from build123d import *

# Parameters (mm, degrees)
SKETCH_1_W          = 16
SKETCH_1_H          = 26
EXTRUDE_1_DEPTH     = 5
CUT_EXTRUDE_START   = 1
SKETCH_2_W          = 14
SKETCH_2_H          = 25
CUT_EXTRUDE_1_DEPTH = 10
EXTRUDE_START       = 5
SKETCH_3_W          = 16
SKETCH_3_H          = 26
EXTRUDE_3_DEPTH     = 1
CUT_EXTRUDE_START_2 = 6
SKETCH_4_W          = 14
SKETCH_4_H          = 17
CUT_EXTRUDE_2_DEPTH = 1
SKETCH_6_W          = 16
SKETCH_6_H          = 26
CUT_EXTRUDE_4_DEPTH = 5


with BuildPart() as part:
    # 스케치1 → 보스-돌출1 (new body)
    with BuildSketch(Plane(origin=(0, 0, 0), x_dir=(1, 0, 0), z_dir=(0, 1, 0))):
        Rectangle(SKETCH_1_W, SKETCH_1_H)
    extrude(amount=EXTRUDE_1_DEPTH)

    # 스케치2 → 컷-돌출1 (cut)
    with BuildSketch(Plane(origin=(0, 0, 0), x_dir=(1, 0, 0), z_dir=(0, 1, 0)).offset(CUT_EXTRUDE_START)):
        with Locations((0, 0.5)):
            Rectangle(SKETCH_2_W, SKETCH_2_H)
    extrude(amount=CUT_EXTRUDE_1_DEPTH, mode=Mode.SUBTRACT)

    # 스케치6 → 컷-돌출4 (cut)
    with BuildSketch(Plane.XZ):
        Rectangle(SKETCH_6_W, SKETCH_6_H)
    extrude(amount=-CUT_EXTRUDE_4_DEPTH, mode=Mode.SUBTRACT)


with BuildPart() as body_2:
    # 스케치3 → 보스-돌출3 (new body)
    with BuildSketch(Plane(origin=(0, 0, 0), x_dir=(1, 0, 0), z_dir=(0, 1, 0)).offset(EXTRUDE_START)):
        Rectangle(SKETCH_3_W, SKETCH_3_H)
    extrude(amount=EXTRUDE_3_DEPTH)

    # 스케치4 → 컷-돌출2 (cut)
    with BuildSketch(Plane(origin=(0, 0, 0), x_dir=(1, 0, 0), z_dir=(0, 1, 0)).offset(CUT_EXTRUDE_START_2)):
        with Locations((0, -1.5)):
            Rectangle(SKETCH_4_W, SKETCH_4_H)
    extrude(amount=-CUT_EXTRUDE_2_DEPTH, mode=Mode.SUBTRACT)


solid = body_2.part
For this review, take the finished solid that the model builds, in its own axes (mm). A direction names the side the tool comes from. Round coordinates to 2 decimals unless told otherwise and drop trailing zeros. Order: outer loops, then holes, each group sorted by start corner. A loop starts at its lowest first (then second) coordinate and runs counter-clockwise, first axis right, second up. Notation, with made-up numbers: M 5.25,66 L 41.25,66 A38 cw 41.25,105 Z; hole C 68.5,-26.5 d11. An arc over 180 degrees is marked long. Write each question's results on one line, items separated by ' | '. Start each with the question number.
1. Add section B-B (z = -0.5). State the section outline as (x, y) points, then the cut area to 3 significant figures.
2. Add section A-A (x = -0.5). State the section outline as (y, z) points.
3. To check wall thickness, follow L1, parallel to Z at x = -1.75, y = 5.4; L2, parallel to X at y = 5.4, z = -5. State the ranges of each line that lie inside material, in increasing order. Write a range as [from, to].
4. Tool access review of faces 1 (the face through (-0.1, 5.5, 13)), 2 (the face through (7, 5.5, 1.6)): name each direction out of +Z, -Z, +X, -X, +Y, -Y from which nothing blocks a thin tool from reaching the whole face with its end or side.
5. Add section C-C (y = 5.7). State the section outline as (x, z) points, then the cut area to 3 significant figures.
6. Draft analysis for pull direction Z (two halves, no side actions). For faces 3 (the face through (-0.1, 5.5, 10)), 4 (the face through (-0.1, 5.5, -13)), 5 (the face through (-7.2, 6, -3.1)), state which applies: pulls with the +Z half, pulls with the -Z half, needs draft (parallel to the pull), parting line crosses it, or undercut.
Output values:
1) outline: M -8,5 L -7,5 L -7,6 L -8,6 Z; M 7,5 L 8,5 L 8,6 L 7,6 Z | area: 2.00 mm^2
2) outline: M 5,-13 L 6,-13 L 6,-7 L 5,-7 Z; M 5,10 L 6,10 L 6,13 L 5,13 Z
3) L1: [-13, -7], [10, 13] | L2: [-8, -7], [7, 8]
4) face 1: +Z, +X, -X, +Y, -Y | face 2: +Y, -Y
5) outline: M -8,-13 L 8,-13 L 8,13 L -8,13 Z; hole M -7,-7 L 7,-7 L 7,10 L -7,10 Z | area: 178 mm^2
6) face 3: undercut | face 4: pulls with the -Z half | face 5: needs draft
